Could you check a few things on this model? Use its own coordinates, in mm. Face numbers are marked on the shaded views. A direction names the side the tool comes from. Give positions to 0.01 mm unless a question says otherwise; leave off trailing zeros. Write each loop counter-clockwise with the first axis right and the second up, starting at its lowest first coordinate (ties: lowest second). Pieces come first, ordered by that corner, then holes. Notation, with made-up numbers: (61, 52) - (65, 52) arc R20 ccw to (65, 61) - close; hole circle Ø7 at (54, 75). An arc over 180 degrees is marked (long way). Use one line per item in the form item = value.
```python
from build123d import *

# Parameters (mm, degrees)
BOSS_EXTRU_1_DEPTH = 15
ESQUISSE2_W        = 30
ESQUISSE2_H        = 25
BOSS_EXTRU_2_DEPTH = 5
CONG_1_R           = 0.5


with BuildPart() as part:
    # Esquisse1 → Boss.-Extru.1 (new body)
    with BuildSketch(Plane.XY):
        with BuildLine():
            Line((6, 0), (10, 0))
            Line((10, 0), (10, -100))
            Line((10, -100), (-10, -100))
            Line((-10, -100), (-10, 0))
            Line((-10, 0), (-6, 0))
            ThreePointArc((-6, 0), (0, -6), (6, 0))
        make_face()
    extrude(amount=BOSS_EXTRU_1_DEPTH)

    # Esquisse2 → Boss.-Extru.2 (add)
    with BuildSketch(Plane.XZ.offset(100)):
        with Locations((0, 7.5)):
            Rectangle(ESQUISSE2_W, ESQUISSE2_H)
    extrude(amount=BOSS_EXTRU_2_DEPTH)

    # Congé1
    cong_1_edges = [part.edges().sort_by_distance(p)[0] for p in [
        (10, -50, 15),
        (-10, 0, 7.5),
        (-6, 0, 7.5),
        (6, 0, 7.5),
        (10, 0, 7.5),
        (8, 0, 15),
        (0, -6, 15),
        (-15, -100, 7.5),
        (-8, 0, 15),
        (0, -100, -5),
        (15, -100, 7.5),
        (0, -100, 20),
        (-10, -50, 15),
        (-8, 0, 0),
        (0, -6, 0),
        (8, 0, 0),
        (10, -50, 0),
        (-10, -50, 0),
    ]]
    fillet(cong_1_edges, radius=CONG_1_R)


solid = part.part
```
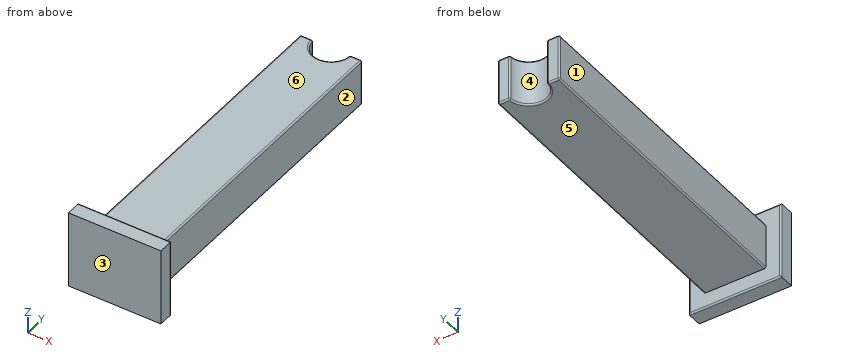
1. Imagine slicing it at C-C, the plane y = -90.5. List the corners of the cut face in (x, z) for me, and give its area (3 significant figures).
Response values:
outline = (-10, 0.5) arc R0.5 ccw to (-9.5, 0) - (9.5, 0) arc R0.5 ccw to (10, 0.5) - (10, 14.5) arc R0.5 ccw to (9.5, 15) - (-9.5, 15) arc R0.5 ccw to (-10, 14.5) - close
area = 300 mm²
2. Imagine slicing it at A-A, the plane x = 0. List the corners of the cut face in (y, z) for me, and give its area (3 significant figures).
Response values:
outline = (-105, -5) - (-100.5, -5) arc R0.5 ccw to (-100, -4.5) - (-100, 0) - (-6.5, 0) arc R0.5 ccw to (-6, 0.5) - (-6, 14.5) arc R0.5 ccw to (-6.5, 15) - (-100, 15) - (-100, 19.5) arc R0.5 ccw to (-100.5, 20) - (-105, 20) - close
area = 1,530 mm²
3. If we mould it in two halves opening along X, with no side actions, what happens to the marked faces 1, 2, 3 and 4? For each: pulls with the +X half, pulls with the -X half, needs draft (parallel to the pull), parting line crosses it, or undercut.
Response values:
face_1 = pulls with the -X half
face_2 = pulls with the +X half
face_3 = needs draft
face_4 = undercut
4. For pin 1 (12 mm diameter, centred on y = -34.5, z = 0, fed in from -X); pin 2 (1 mm diameter, centred on x = -8, y = -69, fed in from -Z); pin 3 (5.5 mm diameter, centred on x = -4.5, y = -69, fed in from +Z), each with a flat end and sliding along its axis, tell me the tip position at first contact or that it passes through.
Response values:
pin_1 = -10
pin_2 = 0
pin_3 = 15
5. Imagine slicing it at B-B, the plane z = 5.5. List the corners of the cut face in (x, y) for me, and give its area (3 significant figures).
Response values:
outline = (-15, -105) - (15, -105) - (15, -100.5) arc R0.5 ccw to (14.5, -100) - (10, -100) - (10, -0.5) arc R0.5 ccw to (9.5, 0) - (6.48, 0) arc R0.5 ccw to (5.98, -0.46) arc R6 cw to (-5.98, -0.46) arc R0.5 ccw to (-6.48, 0) - (-9.5, 0) arc R0.5 ccw to (-10, -0.5) - (-10, -100) - (-14.5, -100) arc R0.5 ccw to (-15, -100.5) - close
area = 2,090 mm²
6. Which directions (+Z, -Z, +X, -X, +Y, -Y) give clear straight access to the entire face, cutting with the end or side of a thin tool? Please do the marked faces 5 and 6.
Response values:
face_5 = -Z, +X, -X, +Y
face_6 = +Z, +X, -X, +Y
7. If I drill on line 1 (Z direction, x = 5.5, y = -45.5); line 2 (X direction, y = -52, z = 6.5); line 3 (Y direction, x = -0.25, z = 3.5), over which ranges is the centre line in solid material (lowest first)? Write a range as from..to.
Response values:
line_1 = 0..15
line_2 = -10..10
line_3 = -105..-5.99
8. Imagine slicing it at D-D, the plane z = -2. List the corners of the cut face in (x, y) for me.
Response values:
outline = (-15, -105) - (15, -105) - (15, -100.5) arc R0.5 ccw to (14.5, -100) - (-14.5, -100) arc R0.5 ccw to (-15, -100.5) - close
